Build history of the part. All positions in model axes, mm. A direction names the side the tool comes from. Give positions to 0.01 mm unless a question says otherwise; leave off trailing zeros. Write each loop counter-clockwise with the first axis right and the second up, starting at its lowest first coordinate (ties: lowest second). Pieces come first, ordered by that corner, then holes.
from build123d import *

# Parameters (mm, degrees)
SKETCH1_R           = 9.2
BOSS_EXTRUDE1_DEPTH = 8.2
BOSS_EXTRUDE2_DEPTH = 1.8


with BuildPart() as part:
    # Sketch1 → Boss-Extrude1 (new body)
    with BuildSketch(Plane(origin=(0, 0, 0), x_dir=(1, 0, 0), z_dir=(0, 1, 0))):
        with BuildLine():
            Line((-9.1, 10.1), (-7, 10.1))
            Line((-7, 10.1), (-7.5, 8.7))
            Line((-7.5, 8.7), (-4.5, 8.7))
            Line((-4.5, 8.7), (-5, 10.1))
            Line((-5, 10.1), (5, 10.1))
            Line((5, 10.1), (4.5, 8.7))
            Line((4.5, 8.7), (7.5, 8.7))
            Line((7.5, 8.7), (7, 10.1))
            Line((7, 10.1), (9.1, 10.1))
            ThreePointArc((9.1, 10.1), (9.807106781, 9.807106781), (10.1, 9.1))
            Line((10.1, 9.1), (10.1, 7))
            Line((10.1, 7), (8.7, 7.5))
            Line((8.7, 7.5), (8.7, 4.5))
            Line((8.7, 4.5), (10.1, 5))
            Line((10.1, 5), (10.1, -5))
            Line((10.1, -5), (8.7, -4.5))
            Line((8.7, -4.5), (8.7, -7.5))
            Line((8.7, -7.5), (10.1, -7))
            Line((10.1, -7), (10.1, -9.1))
            ThreePointArc((10.1, -9.1), (9.807106781, -9.807106781), (9.1, -10.1))
            Line((9.1, -10.1), (7, -10.1))
            Line((7, -10.1), (7.5, -11.5))
            Line((7.5, -11.5), (4.5, -11.5))
            Line((4.5, -11.5), (5, -10.1))
            Line((5, -10.1), (-5, -10.1))
            Line((-5, -10.1), (-4.5, -11.5))
            Line((-4.5, -11.5), (-7.5, -11.5))
            Line((-7.5, -11.5), (-7, -10.1))
            Line((-7, -10.1), (-9.1, -10.1))
            ThreePointArc((-9.1, -10.1), (-9.807106781, -9.807106781), (-10.1, -9.1))
            Line((-10.1, -9.1), (-10.1, -7))
            Line((-10.1, -7), (-11.5, -7.5))
            Line((-11.5, -7.5), (-11.5, -4.5))
            Line((-11.5, -4.5), (-10.1, -5))
            Line((-10.1, -5), (-10.1, 5))
            Line((-10.1, 5), (-11.5, 4.5))
            Line((-11.5, 4.5), (-11.5, 7.5))
            Line((-11.5, 7.5), (-10.1, 7))
            Line((-10.1, 7), (-10.1, 9.1))
            ThreePointArc((-10.1, 9.1), (-9.807106781, 9.807106781), (-9.1, 10.1))
        make_face()
        Circle(SKETCH1_R, mode=Mode.SUBTRACT)
    extrude(amount=BOSS_EXTRUDE1_DEPTH)

    # Sketch2 → Boss-Extrude2 (add)
    with BuildSketch(Plane(origin=(0, 8.2, 0), x_dir=(1, 0, 0), z_dir=(0, 1, 0))):
        with BuildLine():
            Line((-9.1, 4), (-5, 4))
            ThreePointArc((-5, 4), (-4.292893219, 4.292893219), (-4, 5))
            Line((-4, 5), (-4, 9.1))
            ThreePointArc((-4, 9.1), (-4.292893219, 9.807106781), (-5, 10.1))
            Line((-5, 10.1), (-9.1, 10.1))
            ThreePointArc((-9.1, 10.1), (-9.807106781, 9.807106781), (-10.1, 9.1))
            Line((-10.1, 9.1), (-10.1, 5))
            ThreePointArc((-10.1, 5), (-9.807106781, 4.292893219), (-9.1, 4))
        make_face()
        with BuildLine():
            Line((10.1, 9.1), (10.1, 5))
            ThreePointArc((10.1, 5), (9.807106781, 4.292893219), (9.1, 4))
            Line((9.1, 4), (5, 4))
            ThreePointArc((5, 4), (4.292893219, 4.292893219), (4, 5))
            Line((4, 5), (4, 9.1))
            ThreePointArc((4, 9.1), (4.292893219, 9.807106781), (5, 10.1))
            Line((5, 10.1), (9.1, 10.1))
            ThreePointArc((9.1, 10.1), (9.807106781, 9.807106781), (10.1, 9.1))
        make_face()
        with BuildLine():
            Line((9.1, -4), (5, -4))
            ThreePointArc((5, -4), (4.292893219, -4.292893219), (4, -5))
            Line((4, -5), (4, -9.1))
            ThreePointArc((4, -9.1), (4.292893219, -9.807106781), (5, -10.1))
            Line((5, -10.1), (9.1, -10.1))
            ThreePointArc((9.1, -10.1), (9.807106781, -9.807106781), (10.1, -9.1))
            Line((10.1, -9.1), (10.1, -5))
            ThreePointArc((10.1, -5), (9.807106781, -4.292893219), (9.1, -4))
        make_face()
        with BuildLine():
            Line((-4, -5), (-4, -9.1))
            ThreePointArc((-4, -9.1), (-4.292893219, -9.807106781), (-5, -10.1))
            Line((-5, -10.1), (-9.1, -10.1))
            ThreePointArc((-9.1, -10.1), (-9.807106781, -9.807106781), (-10.1, -9.1))
            Line((-10.1, -9.1), (-10.1, -5))
            ThreePointArc((-10.1, -5), (-9.807106781, -4.292893219), (-9.1, -4))
            Line((-9.1, -4), (-5, -4))
            ThreePointArc((-5, -4), (-4.292893219, -4.292893219), (-4, -5))
        make_face()
    extrude(amount=BOSS_EXTRUDE2_DEPTH)


solid = part.part
(1) Mould opens along X. For faces 6 (the face through (9.39, 4.043, 7.254)), 7 (the face through (-9, 0, 4)), 8 (the face through (9.815, 9.087, 4.301)) say: +X half, -X half, draft (parallel to the pull), parting line (faces both ways), or undercut.
(2) Saw through at D-D, the plane x = -6. List the corners of the cut face in (y, z), plus the area to 3 significant figures.
(3) Saw through at B-B, the plane x = 0. List the corners of the cut face in (y, z), plus the area to 3 significant figures.
(4) Saw through at A-A, the plane z = 0. List the corners of the cut face in (x, y).
(5) Saw through at C-C, the plane z = 5.5. List the corners of the cut face in (x, y).
(6) Probe line 1 (Z direction, x = 0, y = 3.5); line 2 (Z direction, x = -6.5, y = 9.75). List the from-to ranges inside material, lowest first.
(7) 3-axis set-ups, long thin cutter, end or side, ignore diameter. For faces 1 (the face through (4.746, 4.043, 10.81)), 2 (the face through (4.285, 9.087, -9.799)), 3 (the face through (4, 9, 7)), 4 (the face through (-7, 9, -4)), 5 (the face through (-6, 8.2, 6)): which of +Z, -Z, +X, -X, +Y, -Y reach the whole face in a straight line?
(8) Drop flat-ended pins along their axis: pin 1 (1.5 mm diameter, centred on x = 5.5, z = 10.5, fed in from +Y); pin 2 (0.7 mm diameter, centred on x = 9.5, z = -6, fed in from -Y); pin 3 (0.9 mm diameter, centred on x = -6.5, y = 9, fed in from +Z); pin 4 (0.9 mm diameter, centred on y = 3, z = -6, fed in from +X). Give the stop position or say it passes through.
Computed values:
1. face 6: undercut
1. face 7: draft
1. face 8: +X half
2. outline: (0, -8.7) - (8.2, -8.7) - (8.2, -10.1) - (10, -10.1) - (10, -4) - (8.2, -4) - (8.2, -6.97) - (0, -6.97) - close; (0, 6.97) - (8.2, 6.97) - (8.2, 4) - (10, 4) - (10, 10.1) - (8.2, 10.1) - (8.2, 11.5) - (0, 11.5) - close
2. area: 73.2 mm2
3. outline: (0, -10.1) - (8.2, -10.1) - (8.2, -9.2) - (0, -9.2) - close; (0, 9.2) - (8.2, 9.2) - (8.2, 10.1) - (0, 10.1) - close
3. area: 14.8 mm2
4. outline: (-10.1, 0) - (-9.2, 0) - (-9.2, 8.2) - (-10.1, 8.2) - close; (9.2, 0) - (10.1, 0) - (10.1, 8.2) - (9.2, 8.2) - close
5. outline: (-11.5, 0) - (-7.37, 0) - (-7.37, 8.2) - (-4, 8.2) - (-4, 10) - (-10.1, 10) - (-10.1, 8.2) - (-11.5, 8.2) - close; (4, 8.2) - (7.37, 8.2) - (7.37, 0) - (8.7, 0) - (8.7, 8.2) - (10.1, 8.2) - (10.1, 10) - (4, 10) - close
6. line 1: z = -10.1 to -9.2, 9.2 to 10.1
6. line 2: z = -10.1 to -4, 4 to 10.1
7. face 1: +Y, -Y
7. face 2: -Z, +Y
7. face 3: +Z, -Z, +Y
7. face 4: +X, -X, +Y
7. face 5: -Y
8. pin 1: stops at y = 10
8. pin 2: stops at y = 8.2
8. pin 3: stops at z = 10.1
8. pin 4: stops at x = 8.7
